from build123d import *

# Parameters (mm, degrees)
SKETCH1_R               = 9.525
BOSS_EXTRUDE1_DEPTH     = 9.525
SKETCH2_R               = 3.96875
BOSS_EXTRUDE2_DEPTH     = 3.175
FILLET1_R               = 0.79248
BOSS_EXTRUDE3_START     = 3.175
SKETCH3_R               = 3.96875
BOSS_EXTRUDE3_DEPTH     = 3.175
CUT_EXTRUDE1_DEPTH      = 19.513272318
CUT_EXTRUDE1_DEPTH_BACK = 19.513272318
SKETCH13_R              = 4.7625


with BuildPart() as part:
    # Sketch1 → Boss-Extrude1 (new, symmetric)
    with BuildSketch(Plane(origin=(0, 0, 0), x_dir=(0, 0, -1), z_dir=(1, 0, 0))):
        with Locations(Location((0, 0, 0), (0, 0, 180))):
            Circle(SKETCH1_R)
    extrude(amount=BOSS_EXTRUDE1_DEPTH, both=True)

    # Sketch2 → Boss-Extrude2 (add)
    with BuildSketch(Plane(origin=(9.525, 0, 0), x_dir=(0, 0, -1), z_dir=(1, 0, 0))):
        Circle(SKETCH2_R)
    extrude(amount=BOSS_EXTRUDE2_DEPTH)

    # Fillet1
    fillet1_edges = [part.edges().sort_by_distance(p)[0] for p in [
        (-9.525, 0, -9.525),
        (9.525, 0, -9.525),
    ]]
    fillet(fillet1_edges, radius=FILLET1_R)

    # Sketch3 → Boss-Extrude3 (add)
    with BuildSketch(Plane.ZY.offset(9.525).offset(BOSS_EXTRUDE3_START)):
        with Locations(Location((0, 0, 0), (0, 0, 180))):
            Circle(SKETCH3_R)
    extrude(amount=-BOSS_EXTRUDE3_DEPTH)

    # Sketch13 → Cut-Extrude1 (cut, two sides: drawn at the far end of the back side and taken through both)
    with BuildSketch(Plane.XY.offset(-CUT_EXTRUDE1_DEPTH_BACK)):
        with Locations(Location((0, 0, 0), (0, 0, 180))):
            Circle(SKETCH13_R)
    extrude(amount=CUT_EXTRUDE1_DEPTH + CUT_EXTRUDE1_DEPTH_BACK, mode=Mode.SUBTRACT)


solid = part.part
The listing builds one solid part. Answer for the finished solid, in the listing's coordinates (mm). A direction names the side the tool comes from. Round coordinates to 2 decimals unless told otherwise and drop trailing zeros. Order: outer loops, then holes, each group sorted by start corner. A loop starts at its lowest first (then second) coordinate and runs counter-clockwise, first axis right, second up. Notation, with made-up numbers: (77.5, 67) -> (86.5, 67) arc R26 cw to (86.5, 85) -> close; hole circle Ø10 at (-25, 21). An arc over 180 degrees is marked (long way). One line per item, written item: value.
Item 1: Given P1, Ø10, axis at x = 9.5, z = 7, coming from the -Y side; P2, Ø6, axis at x = -3.5, z = 5.5, coming from the -Y side; P3, Ø5, axis at x = 1.5, y = 1, coming from the +Z side; P4, Ø11, axis at x = 0, y = 0, coming from the +Z side (3 decimals), each flat-ended and moving along its own axis, determine where each tip first touches the part or whether it passes through.
Taken from the geometry:
P1: stops at y = -9.3
P2: stops at y = -9.19
P3: passes through
P4: stops at z = 9.525
Item 2: For a pull along X with two mould halves and no side action, classify faces 1 (the cylindrical face through (-2.56, -4.016, -0.133)), 2 (the flat face through (12.7, 0, 0)), 3 (the flat face through (-12.7, 0, 0)) as released by +X, released by -X, zero draft, split by the parting line, or undercut.
Taken from the geometry:
face 1: undercut
face 2: released by +X
face 3: released by -X
Item 3: Find section A-A, the plane z = 0. Give the vertices of the cut face in (x, y) (1 decimal), then the cut area to 3 significant figures.
Taken from the geometry:
outline: (-12.7, -4) -> (-9.5, -4) -> (-9.5, -8.7) arc R0.8 ccw to (-8.7, -9.5) -> (8.7, -9.5) arc R0.8 ccw to (9.5, -8.7) -> (9.5, -4) -> (12.7, -4) -> (12.7, 4) -> (9.5, 4) -> (9.5, 8.7) arc R0.8 ccw to (8.7, 9.5) -> (-8.7, 9.5) arc R0.8 ccw to (-9.5, 8.7) -> (-9.5, 4) -> (-12.7, 4) -> close; hole circle Ø9.5 at (0, 0)
area: 342 mm2
Item 4: Straight lines are drawn through the part: L1, parallel to X at y = 3.75, z = -1.5 (3 decimals); L2, parallel to X at y = -0.5, z = -1.25; L3, parallel to X at y = 7.75, z = 4 (3 decimals). For each, find the intervals that lie inside material, in ascending order.
Taken from the geometry:
L1: x = -9.525 to -2.936, 2.936 to 9.525
L2: x = -12.7 to -4.74, 4.74 to 12.7
L3: x = -9.525 to 9.525
Item 5: Find section C-C, the plane x = -6. Give the vertices of the cut face in (y, z) (3 decimals).
Taken from the geometry:
outline: circle Ø19.05 at (0, 0)
Item 6: Find section B-B, the plane x = 3.5. Give the vertices of the cut face in (y, z) (3 decimals), then the cut area to 3 significant figures.
Taken from the geometry:
outline: (-3.23, -8.961) -> (-3.23, 8.961) arc R9.525 ccw to start; (3.23, -8.961) arc R9.525 ccw to (3.23, 8.961) -> close
area: 164 mm2
Item 7: For faces 4 (the cylindrical face through (-11.135, 3.874, 0.86)), 5 (the flat face through (9.525, 2, 4)), 6 (the cylindrical face through (0.122, 5.796, -7.559)), determine the directions among +Z, -Z, +X, -X, +Y, -Y from which every point of the face is accessible in a straight line to the end or side of a thin tool.
Taken from the geometry:
face 4: -X
face 5: +X
face 6: +X, -X
